Check sheet for the modelled part. Datum: model origin and axes. Units: mm. A direction names the side the tool comes from. Give positions to 0.01 mm unless a question says otherwise; leave off trailing zeros. Loops run counter-clockwise (first coordinate to the right, second up) from the corner with the lowest first, then second, coordinate; pieces in that order, holes last.
```python
from build123d import *

# Parameters (mm, degrees)
EXTRUDE_1_DEPTH        = 820
SKETCH_2_W             = 10
SKETCH_2_H             = 10
EXTRUDE_2_DEPTH        = 20
SKETCH_4_W             = 20
SKETCH_4_H             = 20
EXTRUDE_3_DEPTH        = 10
SKETCH_5_W             = 10
SKETCH_5_H             = 10
CUT_EXTRUDE_2_DEPTH    = 837.973715238
CUT_EXTRUDE_3_DEPTH    = 837.973715238
SKETCH_7_W             = 20
SKETCH_7_H             = 15
CUT_EXTRUDE_4_DEPTH    = 837.973715238
PATTERN_LINEAR_1_COUNT = 6
PATTERN_LINEAR_1_PITCH = 30
SKETCH_8_W             = 20
SKETCH_8_H             = 15
CUT_EXTRUDE_5_DEPTH    = 837.973715238
PATTERN_LINEAR_2_COUNT = 5
PATTERN_LINEAR_2_PITCH = 30


with BuildPart() as part:
    # Эскиз1 → Бобышка-Вытянуть1 (new body)
    with BuildSketch(Plane.XY):
        Polygon((0, 0), (0, 155), (10, 155), (10, 165), (20, 165), (20, 145), (30, 145), (30, 10), (10, 10), (10, 0), align=None)
    extrude(amount=EXTRUDE_1_DEPTH)

    # Эскиз2 → Бобышка-Вытянуть2 (add)
    with BuildSketch(Plane(origin=(10, 0, 0), x_dir=(0, 0, -1), z_dir=(1, 0, 0))):
        with Locations((-815, 5)):
            Rectangle(SKETCH_2_W, SKETCH_2_H)
        with Locations((-5, 5)):
            Rectangle(SKETCH_2_W, SKETCH_2_H)
    extrude(amount=EXTRUDE_2_DEPTH)

    # Эскиз4 → Бобышка-Вытянуть3 (add)
    with BuildSketch(Plane(origin=(20, 0, 0), x_dir=(0, 0, -1), z_dir=(1, 0, 0))):
        with Locations((-810, 155)):
            Rectangle(SKETCH_4_W, SKETCH_4_H)
        with Locations((-10, 155)):
            Rectangle(SKETCH_4_W, SKETCH_4_H)
    extrude(amount=EXTRUDE_3_DEPTH)

    # Эскиз5 → Вырез-Вытянуть2 (cut, through all)
    with BuildSketch(Plane(origin=(30, 0, 0), x_dir=(0, 0, -1), z_dir=(1, 0, 0))):
        with Locations((-815, 160)):
            Rectangle(SKETCH_5_W, SKETCH_5_H)
        with Locations((-5, 160)):
            Rectangle(SKETCH_5_W, SKETCH_5_H)
    extrude(amount=-CUT_EXTRUDE_2_DEPTH, mode=Mode.SUBTRACT)

    # Эскиз6 → Вырез-Вытянуть3 (cut, through all)
    with BuildSketch(Plane(origin=(30, 0, 0), x_dir=(0, 0, -1), z_dir=(1, 0, 0))):
        with BuildLine():
            Line((-155, 91.846489001), (-255, 91.846489001))
            ThreePointArc((-255, 91.846489001), (-259, 95.846489001), (-255, 99.846489001))
            Line((-255, 99.846489001), (-155, 99.846489001))
            ThreePointArc((-155, 99.846489001), (-151, 95.846489001), (-155, 91.846489001))
        make_face()
        with BuildLine():
            Line((-665, 99.846489001), (-565, 99.846489001))
            ThreePointArc((-565, 99.846489001), (-561, 95.846489001), (-565, 91.846489001))
            Line((-565, 91.846489001), (-665, 91.846489001))
            ThreePointArc((-665, 91.846489001), (-669, 95.846489001), (-665, 99.846489001))
        make_face()
    extrude(amount=-CUT_EXTRUDE_3_DEPTH, mode=Mode.SUBTRACT)

    # Эскиз7 → Вырез-Вытянуть4 (cut, through all)
    with BuildSketch(Plane.ZY):
        with Locations((810, 7.5)):
            Rectangle(SKETCH_7_W, SKETCH_7_H)
    cut_extrude_4 = extrude(amount=-CUT_EXTRUDE_4_DEPTH, mode=Mode.SUBTRACT)

    # Линейный массив1: Вырез-Вытянуть4 ×6
    with Locations(*[(0, i * PATTERN_LINEAR_1_PITCH, 0) for i in range(1, PATTERN_LINEAR_1_COUNT)]):
        add(cut_extrude_4, mode=Mode.SUBTRACT)

    # Эскиз8 → Вырез-Вытянуть5 (cut, through all)
    with BuildSketch(Plane.ZY):
        with Locations((10, 22.5)):
            Rectangle(SKETCH_8_W, SKETCH_8_H)
    cut_extrude_5 = extrude(amount=-CUT_EXTRUDE_5_DEPTH, mode=Mode.SUBTRACT)

    # Линейный массив2: Вырез-Вытянуть5 ×5
    with Locations(*[(0, i * PATTERN_LINEAR_2_PITCH, 0) for i in range(1, PATTERN_LINEAR_2_COUNT)]):
        add(cut_extrude_5, mode=Mode.SUBTRACT)


solid = part.part
```
(1) Access from +Z, -Z, +X, -X, +Y, -Y to the whole of each face (thin tool, end or side, straight path). Record for faces 4 (the face through (15, 91.846, 204)), 5 (the face through (15, 15, 10)), 6 (the face through (15, 127, 800)).
(2) Gauge pin test, flat ends, axial feed: pin 1 Ø16.5 at (x, y) = (18, 127.5) entering from +Z; pin 2 Ø2 at (x, z) = (15, 624) entering from -Y; pin 3 Ø12 at (x, y) = (11, 5.5) entering from +Z; pin 4 Ø10 at (x, z) = (13, 808.5) entering from -Y. Record the tip position at first contact, or that the pin passes through.
(3) Release check for a two-part mould opening along Y. For faces 1 (the face through (15, 112, 820)), 2 (the face through (15, 60, 810)), 3 (the face through (15, 15, 810)) record: pulls with the +Y half, pulls with the -Y half, needs draft (parallel to the pull), parting line crosses it, or undercut.
(4) Material ranges on line 1 (Y direction, x = 14.5, z = 602.5); line 2 (Y direction, x = 1.5, z = 581); line 3 (Y direction, x = 14.5, z = 673), recorded low to high.
(5) Section check A-A on z = 435. Record the boundary of the cut face in (x, y), plus the area to 3 significant figures.
(6) Section check B-B on y = 82. Record the boundary of the cut face in (x, z), plus the area to 3 significant figures.
Computed values:
1. face 4: +X, -X
1. face 5: -Z, +X, -X
1. face 6: +Z, +X, -X
2. pin 1: stops at z = 820
2. pin 2: stops at y = 10
2. pin 3: stops at z = 800
2. pin 4: stops at y = 15
3. face 1: needs draft
3. face 2: undercut
3. face 3: pulls with the -Y half
4. line 1: y = 10 to 91.85, 99.85 to 165
4. line 2: y = 0 to 91.85, 99.85 to 155
4. line 3: y = 10 to 165
5. outline: (0, 0) - (10, 0) - (10, 10) - (30, 10) - (30, 145) - (20, 145) - (20, 165) - (10, 165) - (10, 155) - (0, 155) - close
5. area: 4,450 mm2
6. outline: (0, 20) - (30, 20) - (30, 820) - (0, 820) - close
6. area: 24,000 mm2
